Part model, mm, in its own coordinate system. A direction names the side the tool comes from. Coordinates: 2 decimals unless noted, no trailing zeros. Loops run counter-clockwise (first coordinate to the right, second up) from the corner with the lowest first, then second, coordinate; pieces in that order, holes last. Notation, with made-up numbers: (35, 74.25) - (84, 74.25) arc R23 ccw to (84, 86.25) - close; hole circle Ø4 at (13.25, 56.5). An arc over 180 degrees is marked (long way). Use a Markdown table: item, result. Add a question column.
1) Tool access for faces 1 (the face through (2.835, 39.44, 17.003)), 2 (the face through (-2.441, 39.44, 29.516)), 3 (the face through (10.857, 39, 20)): list every direction of +Z, -Z, +X, -X, +Y, -Y with a clear straight run to the whole face (end or side of a thin tool).
2) Drop flat-ended pins along their axis: P1, Ø2, axis at y = 14.5, z = 19.5, coming from the -X side; P2, Ø2, axis at x = 6.5, y = 51.5, coming from the -Z side. Give the stop position or say it passes through.
3) Pull direction X, two halves, no side cores. Call faces 4 (the face through (16.4, 39.4, 10.7)), 5 (the face through (3.057, 39, 20)), 6 (the face through (1.112, 39.44, 14.948)): +X half, -X half, draft (parallel to the pull), parting line (faces both ways), or undercut.
4) Probe probe 1 along Z at (x, y) = (4, 20.5); probe 2 along X at (y, z) = (14, 23.5); probe 3 along X at (y, z) = (52, 24.5). List the from-to ranges inside material, lowest first. Write a range as [from, to].
5) Band-saw the part on A-A (z = 21). Give the cut face in (x, y), plus the area to 3 significant figures.
from build123d import *

# Parameters (mm, degrees)
EXTRUDE_1_DEPTH = 80


with BuildPart() as part:
    # 草图1 → 凸台-拉伸1 (new body)
    with BuildSketch(Plane(origin=(0, 0, 0), x_dir=(1, 0, 0), z_dir=(0, 1, 0))):
        with BuildLine():
            Line((-1.042752475, -10.085861632), (3.857247525, -10.085861632))
            ThreePointArc((3.857247525, -10.085861632), (4.757247525, -10.985861632), (3.857247525, -11.885861632))
            Line((3.857247525, -11.885861632), (1.076161722, -11.885861632))
            ThreePointArc((1.076161722, -11.885861632), (0.722608332, -12.032308241), (0.576161722, -12.385861632))
            Line((0.576161722, -12.385861632), (0.576161722, -12.790788968))
            ThreePointArc((0.576161722, -12.790788968), (0.614221956, -12.982130685), (0.722608332, -13.144342359))
            Line((0.722608332, -13.144342359), (2.885447948, -15.307181975))
            ThreePointArc((2.885447948, -15.307181975), (3.858717994, -15.957500229), (5.006768291, -16.185861632))
            Line((5.006768291, -16.185861632), (8.907726758, -16.185861632))
            ThreePointArc((8.907726758, -16.185861632), (10.055777055, -15.957500229), (11.029047102, -15.307181975))
            Line((11.029047102, -15.307181975), (13.191886718, -13.144342359))
            ThreePointArc((13.191886718, -13.144342359), (13.300273094, -12.982130685), (13.338333327, -12.790788968))
            Line((13.338333327, -12.790788968), (13.338333327, -12.385861632))
            ThreePointArc((13.338333327, -12.385861632), (13.191886718, -12.032308241), (12.838333327, -11.885861632))
            Line((12.838333327, -11.885861632), (10.057247525, -11.885861632))
            ThreePointArc((10.057247525, -11.885861632), (9.157247525, -10.985861632), (10.057247525, -10.085861632))
            Line((10.057247525, -10.085861632), (14.957247525, -10.085861632))
            ThreePointArc((14.957247525, -10.085861632), (16.371461087, -10.671648069), (16.957247525, -12.085861632))
            Line((16.957247525, -12.085861632), (16.957247525, -16.985861632))
            ThreePointArc((16.957247525, -16.985861632), (16.057247525, -17.885861632), (15.157247525, -16.985861632))
            Line((15.157247525, -16.985861632), (15.157247525, -14.204775829))
            ThreePointArc((15.157247525, -14.204775829), (15.010800915, -13.851222438), (14.657247525, -13.704775829))
            Line((14.657247525, -13.704775829), (14.252320188, -13.704775829))
            ThreePointArc((14.252320188, -13.704775829), (14.060978472, -13.742836063), (13.898766797, -13.851222438))
            Line((13.898766797, -13.851222438), (11.735927181, -16.014062054))
            ThreePointArc((11.735927181, -16.014062054), (11.085608927, -16.987332101), (10.857247525, -18.135382398))
            Line((10.857247525, -18.135382398), (10.857247525, -22.036340865))
            ThreePointArc((10.857247525, -22.036340865), (11.085608927, -23.184391162), (11.735927181, -24.157661209))
            Line((11.735927181, -24.157661209), (13.898766797, -26.320500825))
            ThreePointArc((13.898766797, -26.320500825), (14.060978472, -26.4288872), (14.252320188, -26.466947434))
            Line((14.252320188, -26.466947434), (14.657247525, -26.466947434))
            ThreePointArc((14.657247525, -26.466947434), (15.010800915, -26.320500825), (15.157247525, -25.966947434))
            Line((15.157247525, -25.966947434), (15.157247525, -23.185861632))
            ThreePointArc((15.157247525, -23.185861632), (16.057247525, -22.285861632), (16.957247525, -23.185861632))
            Line((16.957247525, -23.185861632), (16.957247525, -28.085861632))
            ThreePointArc((16.957247525, -28.085861632), (16.371461087, -29.500075194), (14.957247525, -30.085861632))
            Line((14.957247525, -30.085861632), (10.057247525, -30.085861632))
            ThreePointArc((10.057247525, -30.085861632), (9.157247525, -29.185861632), (10.057247525, -28.285861632))
            Line((10.057247525, -28.285861632), (12.838333327, -28.285861632))
            ThreePointArc((12.838333327, -28.285861632), (13.191886718, -28.139415022), (13.338333327, -27.785861632))
            Line((13.338333327, -27.785861632), (13.338333327, -27.380934295))
            ThreePointArc((13.338333327, -27.380934295), (13.300273094, -27.189592579), (13.191886718, -27.027380904))
            Line((13.191886718, -27.027380904), (11.029047102, -24.864541288))
            ThreePointArc((11.029047102, -24.864541288), (10.055777055, -24.214223034), (8.907726758, -23.985861632))
            Line((8.907726758, -23.985861632), (5.006768291, -23.985861632))
            ThreePointArc((5.006768291, -23.985861632), (3.858717994, -24.214223034), (2.885447948, -24.864541288))
            Line((2.885447948, -24.864541288), (0.722608332, -27.027380904))
            ThreePointArc((0.722608332, -27.027380904), (0.614221956, -27.189592579), (0.576161722, -27.380934295))
            Line((0.576161722, -27.380934295), (0.576161722, -27.785861632))
            ThreePointArc((0.576161722, -27.785861632), (0.722608332, -28.139415022), (1.076161722, -28.285861632))
            Line((1.076161722, -28.285861632), (3.857247525, -28.285861632))
            ThreePointArc((3.857247525, -28.285861632), (4.757247525, -29.185861632), (3.857247525, -30.085861632))
            Line((3.857247525, -30.085861632), (-1.042752475, -30.085861632))
            ThreePointArc((-1.042752475, -30.085861632), (-2.456966038, -29.500075194), (-3.042752475, -28.085861632))
            Line((-3.042752475, -28.085861632), (-3.042752475, -23.185861632))
            ThreePointArc((-3.042752475, -23.185861632), (-2.142752475, -22.285861632), (-1.242752475, -23.185861632))
            Line((-1.242752475, -23.185861632), (-1.242752475, -25.966947434))
            ThreePointArc((-1.242752475, -25.966947434), (-1.096305866, -26.320500825), (-0.742752475, -26.466947434))
            Line((-0.742752475, -26.466947434), (-0.337825138, -26.466947434))
            ThreePointArc((-0.337825138, -26.466947434), (-0.146483422, -26.4288872), (0.015728252, -26.320500825))
            Line((0.015728252, -26.320500825), (2.178567868, -24.157661209))
            ThreePointArc((2.178567868, -24.157661209), (2.828886122, -23.184391162), (3.057247525, -22.036340865))
            Line((3.057247525, -22.036340865), (3.057247525, -18.135382398))
            ThreePointArc((3.057247525, -18.135382398), (2.828886122, -16.987332101), (2.178567868, -16.014062054))
            Line((2.178567868, -16.014062054), (0.015728252, -13.851222438))
            ThreePointArc((0.015728252, -13.851222438), (-0.146483422, -13.742836063), (-0.337825138, -13.704775829))
            Line((-0.337825138, -13.704775829), (-0.742752475, -13.704775829))
            ThreePointArc((-0.742752475, -13.704775829), (-1.096305866, -13.851222438), (-1.242752475, -14.204775829))
            Line((-1.242752475, -14.204775829), (-1.242752475, -16.985861632))
            ThreePointArc((-1.242752475, -16.985861632), (-2.142752475, -17.885861632), (-3.042752475, -16.985861632))
            Line((-3.042752475, -16.985861632), (-3.042752475, -12.085861632))
            ThreePointArc((-3.042752475, -12.085861632), (-2.456966038, -10.671648069), (-1.042752475, -10.085861632))
        make_face()
    extrude(amount=EXTRUDE_1_DEPTH)


solid = part.part
Answer block:
| question | item | result |
|---|---|---|
| 1 | face 1 | +Y, -Y |
| 1 | face 2 | +Z, -X, +Y, -Y |
| 1 | face 3 | +X, +Y, -Y |
| 2 | P1 | x = 3.06 |
| 2 | P2 | z = 16.19 |
| 3 | face 4 | +X half |
| 3 | face 5 | -X half |
| 3 | face 6 | undercut |
| 4 | probe 1 | [10.1, 11.87], [16.01, 24.16], [28.3, 30.07] |
| 4 | probe 2 | [-3.04, -1.24], [2.68, 11.24], [15.16, 16.96] |
| 4 | probe 3 | [-3.04, -1.24], [1.84, 3.33], [10.59, 12.08], [15.16, 16.96] |
| 5 | outline | (3.06, 0) - (10.86, 0) - (10.86, 80) - (3.06, 80) - close |
| 5 | area | 624 mm2 |
